Model file for the job. Use its own axes, mm. Face numbers are marked on the shaded views. A direction names the side the tool comes from. Coordinates: 2 decimals unless noted, no trailing zeros. Order: outer loops, then holes, each group sorted by start corner. A loop starts at its lowest first (then second) coordinate and runs counter-clockwise, first axis right, second up.
from build123d import *

# Parameters (mm, degrees)
CYLINDER_R         = 14
CYLINDER_DEPTH     = 100
POLARPATTERN_COUNT = 3


with BuildPart() as part:
    # Sketch → Revolution (revolve)
    with BuildSketch(Plane.XZ):
        Polygon((4.7, 0), (20, 0), (20, 40), (17, 40), (17, 3), (4.7, 3), align=None)
    revolve(axis=Axis((0, 0, 0), (0, 0, 1)))

    # Cylinder → Cylinder (cut)
    with BuildSketch(Plane(origin=(0, 0, 20), x_dir=(0, 1, 0), z_dir=(1, 0, 0))):
        Circle(CYLINDER_R)
    cylinder = extrude(amount=CYLINDER_DEPTH, mode=Mode.SUBTRACT)

    # PolarPattern: Cylinder ×3 about axis
    polarpattern_axis = Axis((0, 0, 0), (0, 0, 1))
    for i in range(1, POLARPATTERN_COUNT):
        add(cylinder.rotate(polarpattern_axis, i * 360 / POLARPATTERN_COUNT), mode=Mode.SUBTRACT)


solid = part.part
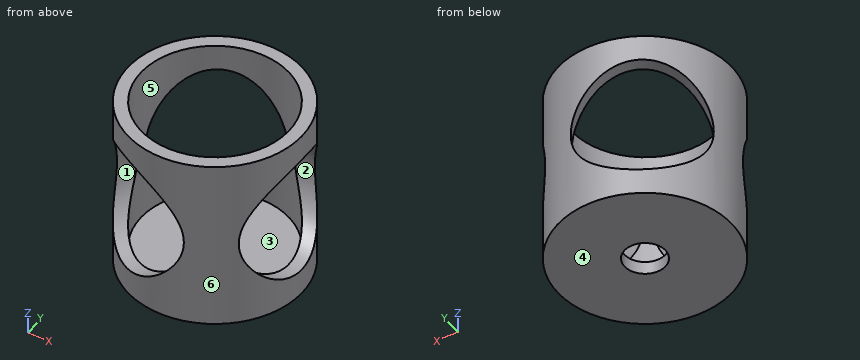
Q1. Mould opens along Y. For the marked faces 4, 5 and 6 say: pulls with the +Y half, pulls with the -Y half, needs draft (parallel to the pull), parting line crosses it, or undercut.
Established:
face 4: needs draft
face 5: undercut
face 6: parting line crosses it
Q2. Probe line 1 (Z direction, x = -11, y = 5); line 2 (Z direction, x = -13, y = -12); line 3 (Y direction, x = 0, z = 2). List the from-to ranges inside material, lowest first.
Established:
line 1: z = 0 to 3
line 2: z = 0 to 7.03, 32.97 to 40
line 3: y = -20 to -4.7, 4.7 to 20
Q3. Cut at C-C, the plane x = 0. Count the separate pieces of the cut face and the enclosed holes in it, plus the area to 3 significant figures.
Established:
separate pieces: 4
enclosed holes: 0
area: 188 mm2
Q4. Cut at B-B, the plane z = 24.5. List the corners of the cut face in (x, y).
Established:
outline: (-18.97, -6.34) - (-16.8, -2.59) arc R17 cw to (-16.8, 2.59) - (-18.97, 6.34) arc R20 ccw to start; (3.99, -19.6) arc R20 ccw to (14.97, -13.26) - (10.64, -13.26) arc R17 cw to (6.16, -15.84) - close; (3.99, 19.6) - (6.16, 15.84) arc R17 cw to (10.64, 13.26) - (14.97, 13.26) arc R20 ccw to start
Q5. Cut at A-A, the plane y = 0. List the corners of the cut face in (x, z).
Established:
outline: (-20, 0) - (-4.7, 0) - (-4.7, 3) - (-17, 3) - (-17, 40) - (-20, 40) - close; (4.7, 0) - (20, 0) - (20, 6) - (17, 6) - (17, 3) - (4.7, 3) - close; (17, 34) - (20, 34) - (20, 40) - (17, 40) - close
Q6. Drop flat-ended pins along their axis: P1, Ø12, axis at x = 11, z = 27, coming from the +Y side; P2, Ø5, axis at y = 3, z = 4.5, coming from the -X side; P3, Ø12, axis at x = 0, y = 0, coming from the +Z side; P4, Ø8, axis at x = -10.5, z = 23, coming from the +Y side. Give the stop position or say it passes through.
Established:
P1: stops at y = 19.36
P2: stops at x = -19.99
P3: stops at z = 3
P4: passes through
Q7. Cut at D-D, the plane z = 19. List the corners of the cut face in (x, y), plus the area to 3 significant figures.
Established:
outline: (-19.25, -5.42) - (-16.94, -1.41) arc R17 cw to (-16.94, 1.41) - (-19.25, 5.42) arc R20 ccw to start; (4.93, -19.38) arc R20 ccw to (14.32, -13.96) - (9.7, -13.96) arc R17 cw to (7.25, -15.38) - close; (4.93, 19.38) - (7.25, 15.38) arc R17 cw to (9.7, 13.96) - (14.32, 13.96) arc R20 ccw to start
area: 63.3 mm2
Q8. Which spindle directions (+Z, -Z, +X, -X, +Y, -Y) get a long thin tool onto all of the face, cutting with end or side? Do the marked faces 1, 2 and 3. Say none if no direction does.
Established:
face 1: none
face 2: +X
face 3: +Z
